from build123d import *

# Parameters (mm, degrees)
SKETCH2_W           = 180
SKETCH2_H           = 150
BOSS_EXTRUDE1_DEPTH = 3
SKETCH4_R           = 1.5
CUT_EXTRUDE1_DEPTH  = 3
SKETCH5_W           = 30
SKETCH5_H           = 100
CUT_EXTRUDE2_DEPTH  = 3
SKETCH7_W           = 40
SKETCH7_H           = 25
BOSS_EXTRUDE4_DEPTH = 3
SKETCH8_W           = 10
SKETCH8_H           = 3
CUT_EXTRUDE4_DEPTH  = 10
SKETCH9_W           = 21
SKETCH9_H           = 150
CUT_EXTRUDE5_DEPTH  = 10
SKETCH10_W          = 30
SKETCH10_H          = 10
CUT_EXTRUDE6_DEPTH  = 10


with BuildPart() as part:
    # Sketch2 → Boss-Extrude1 (new body)
    with BuildSketch(Plane(origin=(0, 0, 0), x_dir=(1, 0, 0), z_dir=(0, 1, 0))):
        Rectangle(SKETCH2_W, SKETCH2_H)
    extrude(amount=BOSS_EXTRUDE1_DEPTH)

    # Sketch4 → Cut-Extrude1 (cut)
    with BuildSketch(Plane(origin=(0, 3, 0), x_dir=(1, 0, 0), z_dir=(0, 1, 0))):
        with Locations(Location((-66.5, -62.49, 0), (0, 0, 270))):
            Circle(SKETCH4_R)
        with Locations(Location((-66.5, -37.49, 0), (0, 0, 270))):
            Circle(SKETCH4_R)
        with Locations(Location((-33.5, -62.49, 0), (0, 0, 90))):
            Circle(SKETCH4_R)
        with Locations(Location((-33.5, -37.49, 0), (0, 0, 90))):
            Circle(SKETCH4_R)
        with Locations(Location((-66.5, 62.49, 0), (0, 0, 90))):
            Circle(SKETCH4_R)
        with Locations(Location((-66.5, 37.49, 0), (0, 0, 90))):
            Circle(SKETCH4_R)
        with Locations(Location((-33.5, 62.49, 0), (0, 0, 270))):
            Circle(SKETCH4_R)
        with Locations(Location((-33.5, 37.49, 0), (0, 0, 270))):
            Circle(SKETCH4_R)
        with Locations(Location((66.5, -62.49, 0), (0, 0, 90))):
            Circle(SKETCH4_R)
        with Locations(Location((33.5, -62.49, 0), (0, 0, 270))):
            Circle(SKETCH4_R)
        with Locations(Location((33.5, -37.49, 0), (0, 0, 270))):
            Circle(SKETCH4_R)
        with Locations(Location((66.5, -37.49, 0), (0, 0, 90))):
            Circle(SKETCH4_R)
        with Locations(Location((66.5, 37.49, 0), (0, 0, 270))):
            Circle(SKETCH4_R)
        with Locations(Location((66.5, 62.49, 0), (0, 0, 270))):
            Circle(SKETCH4_R)
        with Locations(Location((33.5, 62.49, 0), (0, 0, 90))):
            Circle(SKETCH4_R)
        with Locations(Location((33.5, 37.49, 0), (0, 0, 90))):
            Circle(SKETCH4_R)
    extrude(amount=-CUT_EXTRUDE1_DEPTH, mode=Mode.SUBTRACT)

    # Sketch5 → Cut-Extrude2 (cut)
    with BuildSketch(Plane.XZ):
        with Locations((90, 0)):
            Rectangle(SKETCH5_W, SKETCH5_H)
    extrude(amount=-CUT_EXTRUDE2_DEPTH, mode=Mode.SUBTRACT)

    # Sketch7 → Boss-Extrude4 (add)
    with BuildSketch(Plane(origin=(0, 3, 0), x_dir=(1, 0, 0), z_dir=(0, 1, 0))):
        with Locations((110, -62.5)):
            Rectangle(SKETCH7_W, SKETCH7_H)
        with Locations((110, 62.5)):
            Rectangle(SKETCH7_W, SKETCH7_H)
    extrude(amount=-BOSS_EXTRUDE4_DEPTH)

    # Sketch8 → Cut-Extrude4 (cut)
    with BuildSketch(Plane(origin=(0, 3, 0), x_dir=(1, 0, 0), z_dir=(0, 1, 0))):
        with Locations((115, 51.5)):
            Rectangle(SKETCH8_W, SKETCH8_H)
        with Locations((95, 51.5)):
            Rectangle(SKETCH8_W, SKETCH8_H)
        with Locations((115, -51.5)):
            Rectangle(SKETCH8_W, SKETCH8_H)
        with Locations((95, -51.5)):
            Rectangle(SKETCH8_W, SKETCH8_H)
    extrude(amount=-CUT_EXTRUDE4_DEPTH, mode=Mode.SUBTRACT)

    # Sketch9 → Cut-Extrude5 (cut)
    with BuildSketch(Plane(origin=(0, 3, 0), x_dir=(1, 0, 0), z_dir=(0, 1, 0))):
        with Locations((-79.5, 0)):
            Rectangle(SKETCH9_W, SKETCH9_H)
    extrude(amount=-CUT_EXTRUDE5_DEPTH, mode=Mode.SUBTRACT)

    # Sketch10 → Cut-Extrude6 (cut)
    with BuildSketch(Plane(origin=(0, 3, 0), x_dir=(1, 0, 0), z_dir=(0, 1, 0))):
        with Locations((0, -62.49)):
            Rectangle(SKETCH10_W, SKETCH10_H)
        with Locations((0, 62.49)):
            Rectangle(SKETCH10_W, SKETCH10_H)
    extrude(amount=-CUT_EXTRUDE6_DEPTH, mode=Mode.SUBTRACT)


solid = part.part
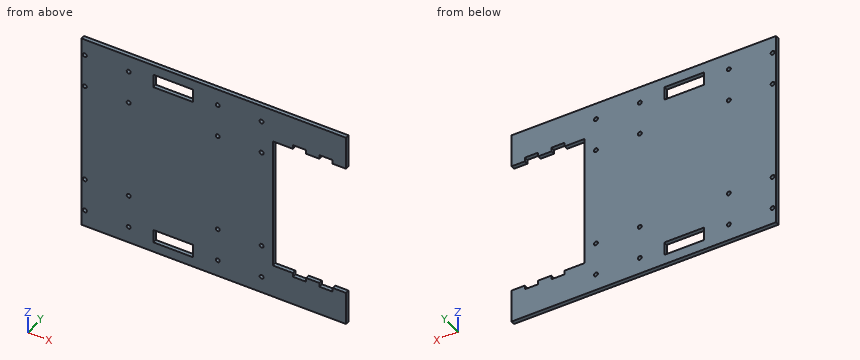
Part model, mm, in its own coordinate system. Coordinates: 2 decimals unless noted, no trailing zeros. Loops run counter-clockwise (first coordinate to the right, second up) from the corner with the lowest first, then second, coordinate; pieces in that order, holes last. Notation, with made-up numbers: (-11.5, 35) -> (30.5, 35) arc R18 cw to (30.5, 59) -> close; hole circle Ø5 at (-11.5, 5.25). An arc over 180 degrees is marked (long way). Use a Markdown table: item, result. Add a question column.
Item 1: Band-saw the part on A-A on x = 77.5. Write the cut outline in (y, z), plus the area to 3 significant figures.
Item 2: Probe probe 1 along X at (y, z) = (2.15, 62.49); probe 2 along X at (y, z) = (1.15, 37.49); probe 3 along Z at (x, y) = (-66.5, 1.4). List the from-to ranges inside material, lowest first.
Item 3: Band-saw the part on B-B on z = -21. Write the cut outline in (x, y), plus the area to 3 significant figures.
Item 4: Band-saw the part on C-C on y = 1.7. Give the number of separate pieces and of enclosed holes in the cut face, plus the area to 3 significant figures.
Geometry says:
| question | item | result |
|---|---|---|
| 1 | outline | (0, -75) -> (3, -75) -> (3, -50) -> (0, -50) -> close; (0, 50) -> (3, 50) -> (3, 75) -> (0, 75) -> close |
| 1 | area | 150 mm² |
| 2 | probe 1 | -69 to -68, -65 to -35, -32 to -15, 15 to 32, 35 to 65, 68 to 130 |
| 2 | probe 2 | -69 to -68, -65 to -35, -32 to 32, 35 to 65, 68 to 75 |
| 2 | probe 3 | -75 to -63.99, -60.99 to -38.99, -35.99 to 35.99, 38.99 to 60.99, 63.99 to 75 |
| 3 | outline | (-69, 0) -> (75, 0) -> (75, 3) -> (-69, 3) -> close |
| 3 | area | 432 mm² |
| 4 | separate pieces | 1 |
| 4 | enclosed holes | 18 |
| 4 | area | 23,500 mm² |
